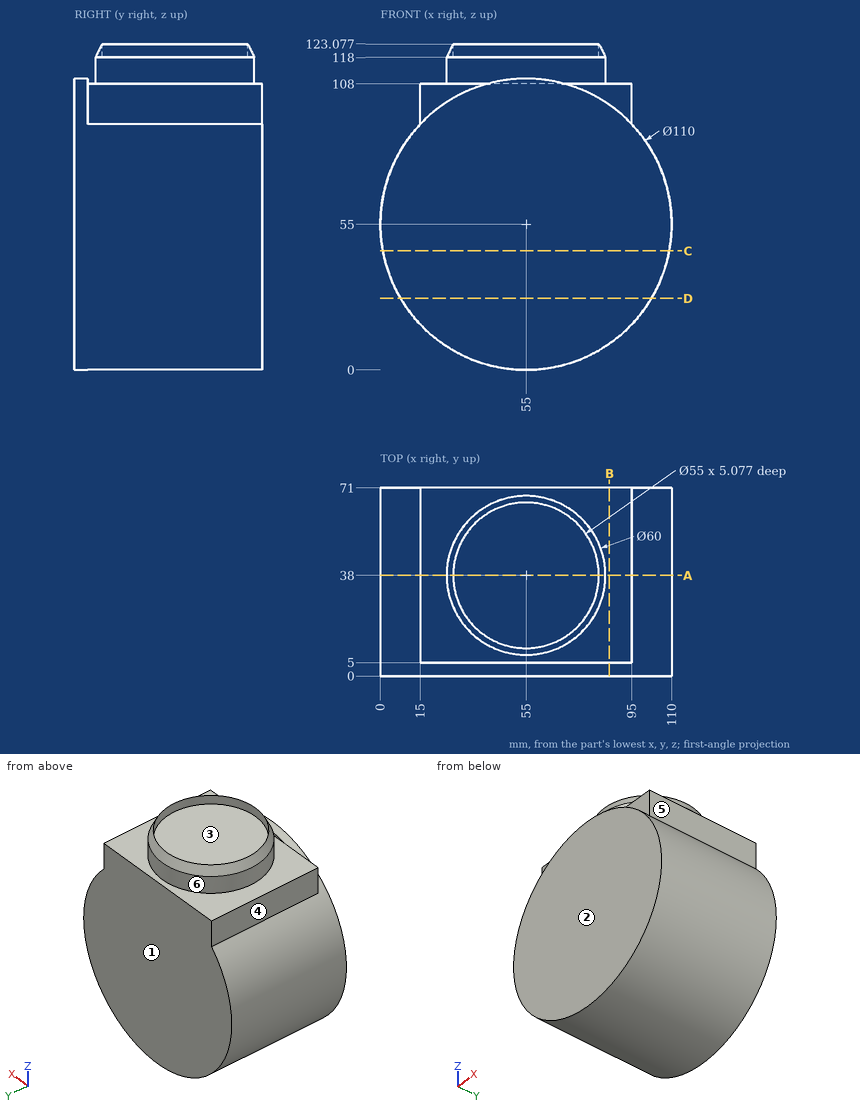
Geometry check sheet. Reference: drawing and pictorial views, mm from the part's lowest x, y, z. A direction names the side the tool comes from. Give positions to 0.01 mm unless a question says otherwise; leave off trailing zeros. Order: outer loops, then holes, each group sorted by start corner. A loop starts at its lowest first (then second) coordinate and runs counter-clockwise, first axis right, second up. Notation, with made-up numbers: M 18,19.25 L 50,19.25 A12 ccw 50,23.25 Z; hole C -19,-24 d4. An arc over 180 degrees is marked long. Answer in a Markdown table with one row per item.
1) Cross-section at B-B, the plane x = 86.5. Enter the section's corners in (y, z).
Filled sheet:
| item | result |
|---|---|
| outline | M 0,9.91 L 71,9.91 L 71,108 L 5,108 L 5,100.09 L 0,100.09 Z |
2) Access from +Z, -Z, +X, -X, +Y, -Y to the whole of each face (thin tool, end or side, straight path). Record for the marked faces 4, 5 and 6.
Filled sheet:
| item | result |
|---|---|
| face 4 | +Z, -X, +Y, -Y |
| face 5 | +Z, +X, +Y, -Y |
| face 6 | +Z |
3) Cross-section at A-A, the plane y = 38. Enter the section's corners in (x, z), plus the area to 3 significant figures.
Filled sheet:
| item | result |
|---|---|
| outline | M 15,92.75 A55 ccw long 95,92.75 L 95,108 L 85,108 L 85,118 L 82.5,123.08 L 82.5,118 L 27.5,118 L 27.5,123.08 L 25,118 L 25,108 L 15,108 Z |
| area | 10,400 mm2 |
4) Cross-section at D-D, the plane z = 27. Enter the section's corners in (x, y), plus the area to 3 significant figures.
Filled sheet:
| item | result |
|---|---|
| outline | M 7.66,0 L 102.34,0 L 102.34,71 L 7.66,71 Z |
| area | 6,720 mm2 |
5) Cross-section at C-C, the plane z = 45. Enter the section's corners in (x, y).
Filled sheet:
| item | result |
|---|---|
| outline | M 0.92,0 L 109.08,0 L 109.08,71 L 0.92,71 Z |
6) Release check for a two-part mould opening along Y. For the marked faces 1, 2 and 3 record: +Y half, -Y half, draft (parallel to the pull), parting line (faces both ways), or undercut.
Filled sheet:
| item | result |
|---|---|
| face 1 | +Y half |
| face 2 | -Y half |
| face 3 | undercut |
7) Thickness scan on L1, parallel to Y at x = 55, z = 120; L2, parallel to Y at x = 91, z = 104.5; L3, parallel to Y at x = 55, z = 120.8. Record the ranges inside material, lowest first. Write a range as [from, to].
Filled sheet:
| item | result |
|---|---|
| L1 | y = [8.98, 10.5], [65.5, 67.02] |
| L2 | y = [5, 71] |
| L3 | y = [9.38, 10.5], [65.5, 66.62] |
8) Gauge pin test, flat ends, axial feed: P1, Ø1.5, axis at y = 59.5, z = 55.5, coming from the -X side; P2, Ø12, axis at y = 37, z = 99.5, coming from the -X side; P3, Ø2, axis at y = 30.5, z = 74.5, coming from the +X side. Record the tip position at first contact, or that the pin passes through.
Filled sheet:
| item | result |
|---|---|
| P1 | stops at x = 0 |
| P2 | stops at x = 15 |
| P3 | stops at x = 106.8 |
